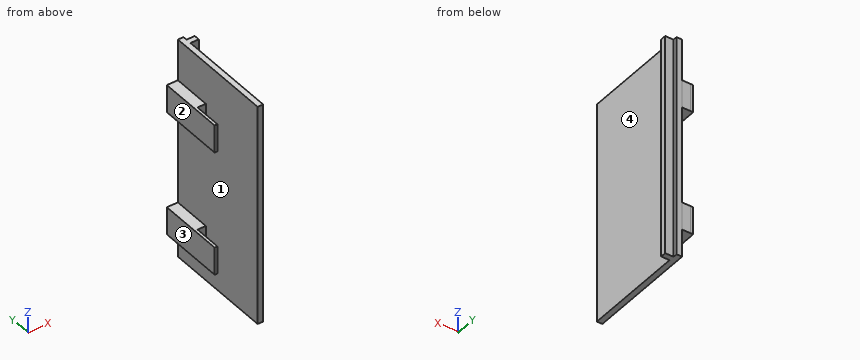
Solid Edge part; units mm, degrees
sketch "Sketch1" plane through (0, 0, 0) normal (-1, 0, 0) x (0, -1, 0)
  line L0 (2.0853, 0) -> (2.0853, 80)
  line L1 (2.0853, 80) -> (-37.9147, 80)
  line L2 (-37.9147, 80) -> (-37.9147, 0)
  line L3 (-37.9147, 0) -> (2.0853, 0)
extrude "Protrusion1" add sketch "Sketch1" against normal blind 2
sketch "Sketch2" plane through (0, 18.9573, 40) normal (-1, 0, 0) x (0, 0, 1)
  line L0 (-20, 4.9573) -> (-20, 18.9573)
  line L1 (-30, 18.9573) -> (-20, 18.9573)
  line L2 (-30, 18.9573) -> (-30, 4.9573)
  line L3 (-30, 4.9573) -> (-20, 4.9573)
  line L4 (25, 18.9573) -> (25, 4.9573)
  line L5 (25, 4.9573) -> (15, 4.9573)
  line L6 (15, 4.9573) -> (15, 18.9573)
  line L7 (15, 18.9573) -> (25, 18.9573)
extrude "Vysunutí_2" add sketch "Sketch2" along normal blind 3
sketch "Sketch3" plane through (-3, 30.9147, 60) normal (-1, 0, 0) x (0, 0, 1)
  line L0 (5, -17) -> (5, 7)
  line L1 (5, 7) -> (-5, 7)
  line L2 (-5, 7) -> (-5, -17)
  line L3 (-5, -17) -> (5, -17)
  line L4 (-40, -17) -> (-40, 7)
  line L5 (-40, 7) -> (-50, 7)
  line L6 (-50, 7) -> (-50, -17)
  line L7 (-50, -17) -> (-40, -17)
extrude "Vysunutí_3" add sketch "Sketch3" along normal blind 1
sketch "Sketch4" plane through (2, 17.9147, 40) normal (1, 0, 0) x (0, 0, 1)
  line L0 (-40, -18.5) -> (40, -18.5)
  line L1 (40, -18.5) -> (40, -16.5)
  line L2 (40, -16.5) -> (-40, -16.5)
extrude "Vysunutí_4" add sketch "Sketch4" along normal blind 3 material side at (2, 36.3647, 40)
Work out the finished part from the listing and answer in its coordinate system (mm). Face numbers are marked on the shaded views. A direction names the side the tool comes from. Give positions to 0.01 mm unless a question says otherwise; leave off trailing zeros. Write each loop counter-clockwise with the first axis right and the second up, starting at its lowest first coordinate (ties: lowest second). Pieces come first, ordered by that corner, then holes. Notation, with made-up numbers: M 70,-2 L 90,-2 A24 cw 90,27 Z; hole C 17.25,-39 d2. An arc over 180 degrees is marked long. Answer as CSV lines item,"result".
Q1. A cutting plane is placed at A-A on y = 22. Write down the section's boundary in (x, z).
A:
outline,"M -4,10 L -3,10 L -3,20 L -4,20 Z; M -4,55 L -3,55 L -3,65 L -4,65 Z; M 0,0 L 2,0 L 2,80 L 0,80 Z"
Q2. A cutting plane is placed at C-C on z = 31. Write down the section's boundary in (x, y), plus the area to 3 significant figures.
A:
outline,"M 0,-2.09 L 2,-2.09 L 2,34.41 L 5,34.41 L 5,36.41 L 2,36.41 L 2,37.91 L 0,37.91 Z"
area,"86.0 mm²"
Q3. A tool of negligible diameter and unlimited length cuts with its end or side. For the marked faces 3 and 4, from which of +Z, -Z, +X, -X, +Y, -Y can it reach the whole face along a straight path? Write none if from no direction.
A:
face 3,"+Z, -Z, -X, +Y, -Y"
face 4,"+Z, -Z, +X, -Y"
Q4. A cutting plane is placed at B-B on x = -0.75. Write down the section's boundary in (y, z), plus the area to 3 significant figures.
A:
outline,"M 23.91,10 L 37.91,10 L 37.91,20 L 23.91,20 Z; M 23.91,55 L 37.91,55 L 37.91,65 L 23.91,65 Z"
area,"280 mm²"
Q5. A cutting plane is placed at D-D on y = 26.5. Write down the section's boundary in (x, z).
A:
outline,"M -4,10 L 0,10 L 0,0 L 2,0 L 2,80 L 0,80 L 0,65 L -4,65 L -4,55 L 0,55 L 0,20 L -4,20 Z"
Q6. The mould has two halves that part along Z. Classify the marked faces 1 and 2: +Z half, -Z half, draft (parallel to the pull), parting line (faces both ways), or undercut.
A:
face 1,"undercut"
face 2,"draft"
Q7. Given P1, Ø18, axis at y = 20.5, z = 57, coming from the +X side; P2, Ø1.5, axis at x = -2, z = 16, coming from the -Y side; P3, Ø0.8, axis at x = -3.5, z = 59.5, coming from the -Y side, each flat-ended and moving along its own axis, determine where each tip first touches the part or whether it passes through.
A:
P1,"stops at x = 2"
P2,"stops at y = 23.91"
P3,"stops at y = 13.91"
Q8. Find the intervals of material crossed by probe 1 along Z at (x, y) = (-2, 34.5); probe 2 along X at (y, z) = (7, 51.5); probe 3 along Y at (x, z) = (4.25, 6), in increasing order. Write a range as [from, to].
A:
probe 1,"z = [10, 20], [55, 65]"
probe 2,"x = [0, 2]"
probe 3,"y = [34.41, 36.41]"
